Geometry check sheet. Reference: the model listing, model coordinates, mm. Face numbers are marked on the shaded views. A direction names the side the tool comes from. Give positions to 0.01 mm unless a question says otherwise; leave off trailing zeros. Loops run counter-clockwise (first coordinate to the right, second up) from the corner with the lowest first, then second, coordinate; pieces in that order, holes last. Notation, with made-up numbers: (-27.75, -21.75) -> (14.25, -21.75) arc R21 cw to (14.25, -2.75) -> close; hole circle Ø5 at (15, 64.25). An arc over 180 degrees is marked (long way). Write item = value, one per line.
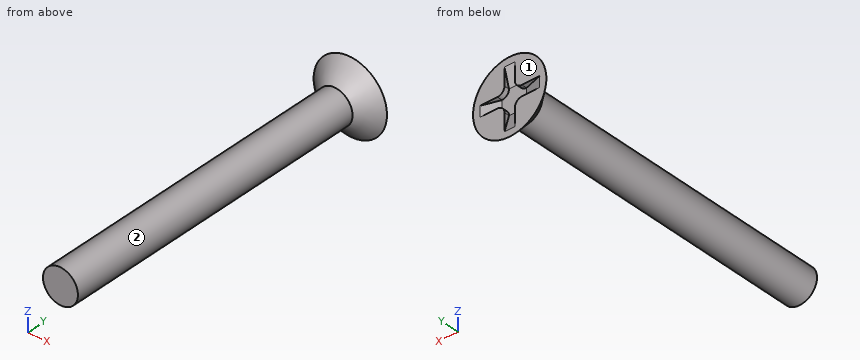
Autodesk Inventor part; units mm, degrees
ref_plane "Work Plane1" through (0, 18, 0) normal (0, 1, 0) x (1, 0, 0)
ref_plane "YZ Plane" through (0, 0, 0) normal (1, 0, 0) x (0, 1, 0)
ref_plane "XZ Plane" through (0, 0, 0) normal (0, 1, 0) x (-1, 0, 0)
sketch "Sketch1" plane through (0, 0, 0) normal (0, 1, 0) x (-1, 0, 0)
  circle A0 centre (0, 0) radius 1
  dimension "d0" = 2
extrude "Extrusion1" add sketch "Sketch1" along normal blind 19
sketch "Sketch2" plane through (0, 19, 0) normal (0, 1, 0) x (1, 0, 0)
  circle A0 centre (0, 0) radius 2.1
  dimension "d3" = 4.2
ref_plane "Work Plane1" through (0, 18, 0) normal (0, 1, 0) x (1, 0, 0)
sketch "Sketch3" plane through (0, 18, 0) normal (0, 1, 0) x (1, 0, 0)
  circle A0 centre (0, 0) radius 1
loft "Loft1" add profiles "Sketch3", "Sketch2"
sketch "Sketch4" plane through (0, 19, 0) normal (0, 1, 0) x (1, 0, 0)
  line L0 (-1.7, -0.3) -> (1.7, -0.3)
  line L1 (1.7, -0.3) -> (1.7, 0.3)
  line L2 (1.7, 0.3) -> (-1.7, 0.3)
  line L3 (-1.7, 0.3) -> (-1.7, -0.3)
  line L4 (-0.3, -1.7) -> (0.3, -1.7)
  line L5 (0.3, -1.7) -> (0.3, 1.7)
  line L6 (0.3, 1.7) -> (-0.3, 1.7)
  line L7 (-0.3, 1.7) -> (-0.3, -1.7)
  point P0 (0, 0)
  point P1 (-1.7, 0)
  point P2 (0, -1.7)
  point P3 (0, -0.3)
  point P4 (0.3, 0)
  point P5 (-0.3, -0.3)
  point P6 (0.3, -0.3)
  point P7 (0.3, 0.3)
  point P8 (-0.3, 0.3)
  dimension "d9" = 3.4
  dimension "d10" = 3.4
  dimension "d11" = 0.6
  dimension "d12" = 0.6
extrude "Extrusion2" cut sketch "Sketch4" against normal blind 0.3
chamfer "Chamfer1" distance 0.3 distance2 1 1 edges at (1.7, 18.7, 0) measured on face at (1.7, 18.9, 0.1)
chamfer "Chamfer2" distance 0.3 distance2 1 1 edges at (0, 18.7, 1.7) measured on face at (-0.1, 18.9, 1.7)
chamfer "Chamfer3" distance 0.3 distance2 1 1 edges at (-1.7, 18.7, 0) measured on face at (-1.7, 18.9, -0.1)
chamfer "Chamfer4" distance 0.3 distance2 1 1 edges at (0, 18.7, -1.7) measured on face at (0.1, 18.9, -1.7)
fillet "Fillet1" radius 0.4 4 edges at (0.3, 18.85, 0.3) (-0.3, 18.85, 0.3) (0.3, 18.85, -0.3) (-0.3, 18.85, -0.3)
thread "Thread1"
equation "\"d12\" = d11"
properties part number "m2_18mm" material "Stainless Steel"
Item 1: Section check B-B, the plane y = 6.5. Record the cut outline in (x, z), plus the area to 3 significant figures.
Answer:
outline = circle Ø2 at (0, 0)
area = 3.14 mm^2
Item 2: Gauge pin test, flat ends, axial feed: pin 1 (2 mm diameter, centred on x = 0.5, z = -0.5, fed in from -Y); pin 2 (0.7 mm diameter, centred on x = 0, z = 0, fed in from +Y). Record the tip position at first contact, or that the pin passes through.
Answer:
pin_1 = 0
pin_2 = 18.7
Item 3: Thickness scan on L1, parallel to Z at x = 0.8, y = 15; L2, parallel to Z at x = -0.35, y = 11; L3, parallel to Y at x = -1.1, z = 0. Record the ranges inside material, lowest first. Write a range as [from, to].
Answer:
L1 = [-0.6, 0.6]
L2 = [-0.94, 0.94]
L3 = [18.09, 18.82]
Item 4: Tool access check on the marked faces 1 and 2. Record the directions out of +Z, -Z, +X, -X, +Y, -Y that give a thin tool (end or side, any length) a straight path to the whole face; none if there is none.
Answer:
face_1 = +Z, -Z, +X, -X, +Y
face_2 = -Y
